Design review of the part built by this model. Coordinates are the model's own, in mm. A direction names the side the tool comes from. Give positions to 0.01 mm unless a question says otherwise; leave off trailing zeros. Order: outer loops, then holes, each group sorted by start corner. A loop starts at its lowest first (then second) coordinate and runs counter-clockwise, first axis right, second up. Notation, with made-up numbers: (61.5, 77.5) -> (119.5, 77.5) arc R13 cw to (119.5, 86.5) -> close; hole circle Ø11 at (31, 34.5). An arc over 180 degrees is marked (long way). Answer in a Markdown table with one row per item. Add a question column.
```python
from build123d import *

# Parameters (mm, degrees)
SKETCH1_W           = 110
SKETCH1_H           = 140
SKETCH1_R           = 2
SKETCH1_R_2         = 2.425
BOSS_EXTRUDE1_DEPTH = 10
FILLET1_R           = 10
SKETCH3_W           = 28.5
SKETCH3_H           = 55
CUT_EXTRUDE1_DEPTH  = 8
CHAMFER1_SIZE       = 8
SKETCH5_R           = 2
CUT_EXTRUDE3_DEPTH  = 8
CUT_EXTRUDE4_START  = -8
SKETCH6_R           = 2
CUT_EXTRUDE4_DEPTH  = 8
SKETCH7_W           = 110
SKETCH7_H           = 15
CUT_EXTRUDE7_DEPTH  = 2.5
CHAMFER3_SIZE       = 2.5
CHAMFER4_SIZE       = 1.5
CUT_EXTRUDE8_DEPTH  = 3
BOSS_EXTRUDE3_DEPTH = 10
SKETCH10_W          = 6.9
SKETCH10_H          = 6.9
CUT_EXTRUDE9_DEPTH  = 5
BOSS_EXTRUDE4_DEPTH = 10


with BuildPart() as part:
    # Sketch1 → Boss-Extrude1 (new body)
    with BuildSketch(Plane.XY):
        Rectangle(SKETCH1_W, SKETCH1_H)
        with Locations((-26.5, 50.75)):
            Circle(SKETCH1_R, mode=Mode.SUBTRACT)
        with Locations(Location((26.5, 50.75, 0), (0, 0, 180))):
            Circle(SKETCH1_R, mode=Mode.SUBTRACT)
        with Locations((26.5, -50.75)):
            Circle(SKETCH1_R, mode=Mode.SUBTRACT)
        with Locations(Location((-26.5, -50.75, 0), (0, 0, 180))):
            Circle(SKETCH1_R, mode=Mode.SUBTRACT)
        with Locations((-40, 55)):
            Circle(SKETCH1_R_2, mode=Mode.SUBTRACT)
        with Locations(Location((40, 55, 0), (0, 0, 180))):
            Circle(SKETCH1_R_2, mode=Mode.SUBTRACT)
        with Locations((40, -55)):
            Circle(SKETCH1_R_2, mode=Mode.SUBTRACT)
        with Locations(Location((-40, -55, 0), (0, 0, 180))):
            Circle(SKETCH1_R_2, mode=Mode.SUBTRACT)
        with Locations((-39.8, 49)):
            Circle(SKETCH1_R_2, mode=Mode.SUBTRACT)
        with Locations(Location((39.8, 49, 0), (0, 0, 180))):
            Circle(SKETCH1_R_2, mode=Mode.SUBTRACT)
        with Locations((39.8, -49)):
            Circle(SKETCH1_R_2, mode=Mode.SUBTRACT)
        with Locations(Location((-39.8, -49, 0), (0, 0, 180))):
            Circle(SKETCH1_R_2, mode=Mode.SUBTRACT)
        with Locations((-39.6, 43.00333426)):
            Circle(SKETCH1_R_2, mode=Mode.SUBTRACT)
        with Locations(Location((39.6, 43.00333426, 0), (0, 0, 180))):
            Circle(SKETCH1_R_2, mode=Mode.SUBTRACT)
        with Locations((39.6, -43.00333426)):
            Circle(SKETCH1_R_2, mode=Mode.SUBTRACT)
        with Locations(Location((-39.6, -43.00333426, 0), (0, 0, 180))):
            Circle(SKETCH1_R_2, mode=Mode.SUBTRACT)
        with BuildLine():
            Line((-7.75, 40), (-7.75, 5))
            ThreePointArc((-7.75, 5), (-9, 3.75), (-10.25, 5))
            Line((-10.25, 5), (-10.25, 40))
            ThreePointArc((-10.25, 40), (-9, 41.25), (-7.75, 40))
        make_face(mode=Mode.SUBTRACT)
        with BuildLine():
            Line((7.75, 40), (7.75, 5))
            ThreePointArc((7.75, 5), (9, 3.75), (10.25, 5))
            Line((10.25, 5), (10.25, 40))
            ThreePointArc((10.25, 40), (9, 41.25), (7.75, 40))
        make_face(mode=Mode.SUBTRACT)
    extrude(amount=BOSS_EXTRUDE1_DEPTH)

    # Fillet1
    fillet1_edges = [part.edges().sort_by_distance(p)[0] for p in [
        (55, -70, 5),
        (-55, -70, 5),
        (-55, 70, 5),
        (55, 70, 5),
    ]]
    fillet(fillet1_edges, radius=FILLET1_R)

    # Sketch3 → Cut-Extrude1 (cut)
    with BuildSketch(Plane.XY.offset(10)):
        with Locations((0, 22.5)):
            Rectangle(SKETCH3_W, SKETCH3_H)
    extrude(amount=-CUT_EXTRUDE1_DEPTH, mode=Mode.SUBTRACT)

    # Chamfer1
    chamfer1_edges = [part.edges().sort_by_distance(p)[0] for p in [
        (0, -5, 10),
        (14.25, 22.5, 10),
        (0, 50, 10),
        (-14.25, 22.5, 10),
    ]]
    chamfer(chamfer1_edges, length=CHAMFER1_SIZE - 0.0001)  # a hair under: the kernel refuses the full size

    # Sketch5 → Cut-Extrude3 (cut)
    with BuildSketch(Plane.ZY.offset(55)):
        with Locations(Location((5, 50, 0), (0, 0, 270))):
            Circle(SKETCH5_R)
        with Locations(Location((5, 40, 0), (0, 0, 270))):
            Circle(SKETCH5_R)
        with Locations(Location((5, 30, 0), (0, 0, 270))):
            Circle(SKETCH5_R)
        with Locations(Location((5, 20, 0), (0, 0, 270))):
            Circle(SKETCH5_R)
        with Locations(Location((5, 10, 0), (0, 0, 270))):
            Circle(SKETCH5_R)
        with Locations(Location((5, 0, 0), (0, 0, 270))):
            Circle(SKETCH5_R)
        with Locations(Location((5, -10, 0), (0, 0, 270))):
            Circle(SKETCH5_R)
        with Locations(Location((5, -20, 0), (0, 0, 270))):
            Circle(SKETCH5_R)
        with Locations(Location((5, -30, 0), (0, 0, 270))):
            Circle(SKETCH5_R)
        with Locations(Location((5, -40, 0), (0, 0, 270))):
            Circle(SKETCH5_R)
        with Locations(Location((5, -50, 0), (0, 0, 270))):
            Circle(SKETCH5_R)
    extrude(amount=-CUT_EXTRUDE3_DEPTH, mode=Mode.SUBTRACT)

    # Sketch6 → Cut-Extrude4 (cut)
    with BuildSketch(Plane(origin=(55, 0, 0), x_dir=(0, 0, -1), z_dir=(1, 0, 0)).offset(CUT_EXTRUDE4_START)):
        with Locations(Location((-5, 50, 0), (0, 0, 270))):
            Circle(SKETCH6_R)
        with Locations(Location((-5, 40, 0), (0, 0, 270))):
            Circle(SKETCH6_R)
        with Locations(Location((-5, 30, 0), (0, 0, 270))):
            Circle(SKETCH6_R)
        with Locations(Location((-5, 20, 0), (0, 0, 270))):
            Circle(SKETCH6_R)
        with Locations(Location((-5, 10, 0), (0, 0, 270))):
            Circle(SKETCH6_R)
        with Locations(Location((-5, 0, 0), (0, 0, 270))):
            Circle(SKETCH6_R)
        with Locations(Location((-5, -10, 0), (0, 0, 270))):
            Circle(SKETCH6_R)
        with Locations(Location((-5, -20, 0), (0, 0, 270))):
            Circle(SKETCH6_R)
        with Locations(Location((-5, -30, 0), (0, 0, 270))):
            Circle(SKETCH6_R)
        with Locations(Location((-5, -40, 0), (0, 0, 270))):
            Circle(SKETCH6_R)
        with Locations(Location((-5, -50, 0), (0, 0, 270))):
            Circle(SKETCH6_R)
    extrude(amount=CUT_EXTRUDE4_DEPTH, mode=Mode.SUBTRACT)

    # Sketch7 → Cut-Extrude7 (cut)
    with BuildSketch(Plane.XY.offset(10)):
        with Locations((0, -15.5)):
            Rectangle(SKETCH7_W, SKETCH7_H)
    extrude(amount=-CUT_EXTRUDE7_DEPTH, mode=Mode.SUBTRACT)

    # Chamfer3
    chamfer3_edges = [part.edges().sort_by_distance(p)[0] for p in [
        (0, -23, 7.5),
        (-37.37495, -8, 7.5),
        (37.37495, -8, 7.5),
    ]]
    chamfer(chamfer3_edges, length=CHAMFER3_SIZE - 0.0001)  # a hair under: the kernel refuses the full size

    # Chamfer4
    chamfer4_edges = [part.edges().sort_by_distance(p)[0] for p in [
        (0, -70, 0),
        (0, -70, 10),
        (55, 0, 0),
        (-55, 0, 0),
        (0, 70, 0),
        (52.071067812, 67.071067812, 0),
        (-52.071067812, 67.071067812, 0),
        (52.071067812, -67.071067812, 0),
        (-52.071067812, -67.071067812, 0),
        (-55, 26, 10),
        (55, -41.5, 10),
        (0, 70, 10),
        (52.071067812, 67.071067812, 10),
        (-52.071067812, 67.071067812, 10),
        (52.071067812, -67.071067812, 10),
        (-52.071067812, -67.071067812, 10),
        (-55, -41.5, 10),
        (55, 26, 10),
    ]]
    chamfer(chamfer4_edges, length=CHAMFER4_SIZE)

    # Sketch8 → Cut-Extrude8 (cut)
    with BuildSketch(Plane(origin=(0, 0, 10), x_dir=(-1, 0, 0), z_dir=(0, 0, -1))):
        with BuildLine():
            Line((-45.8, 43), (-45.8, 55))
            ThreePointArc((-45.8, 55), (-39.8, 61), (-33.8, 55))
            Line((-33.8, 55), (-33.8, 43))
            ThreePointArc((-33.8, 43), (-39.8, 37), (-45.8, 43))
        make_face()
        with BuildLine():
            Line((45.8, 43), (45.8, 55))
            ThreePointArc((45.8, 55), (39.8, 61), (33.8, 55))
            Line((33.8, 55), (33.8, 43))
            ThreePointArc((33.8, 43), (39.8, 37), (45.8, 43))
        make_face()
        with BuildLine():
            Line((45.8, -43), (45.8, -55))
            ThreePointArc((45.8, -55), (39.8, -61), (33.8, -55))
            Line((33.8, -55), (33.8, -43))
            ThreePointArc((33.8, -43), (39.8, -37), (45.8, -43))
        make_face()
        with BuildLine():
            Line((-45.8, -43), (-45.8, -55))
            ThreePointArc((-45.8, -55), (-39.8, -61), (-33.8, -55))
            Line((-33.8, -55), (-33.8, -43))
            ThreePointArc((-33.8, -43), (-39.8, -37), (-45.8, -43))
        make_face()
    extrude(amount=CUT_EXTRUDE8_DEPTH, mode=Mode.SUBTRACT)

    # Sketch9 → Boss-Extrude3 (add)
    with BuildSketch(Plane(origin=(55, 0, 0), x_dir=(0, 0, -1), z_dir=(1, 0, 0))):
        Polygon((-7.479483029, -9.130730638), (-5.687930895, -6.827306465), (-2.453830288, -7.571847612), (-2.453830288, -22.439403639), (-6.432472041, -22.439403639), (-7.150561873, -20.576942606), (-7.150561873, -10.503478378), align=None)
    extrude(amount=-BOSS_EXTRUDE3_DEPTH)

    # Sketch10 → Cut-Extrude9 (cut)
    with BuildSketch(Plane(origin=(0, 0, 0), x_dir=(-1, 0, 0), z_dir=(0, 0, -1))):
        with Locations((-26.5, 50.75)):
            Rectangle(SKETCH10_W, SKETCH10_H)
        with Locations((26.5, 50.75)):
            Rectangle(SKETCH10_W, SKETCH10_H)
        with Locations((26.5, -50.75)):
            Rectangle(SKETCH10_W, SKETCH10_H)
        with Locations((-26.5, -50.75)):
            Rectangle(SKETCH10_W, SKETCH10_H)
    extrude(amount=-CUT_EXTRUDE9_DEPTH, mode=Mode.SUBTRACT)

    # Sketch11 → Boss-Extrude4 (add)
    with BuildSketch(Plane.ZY.offset(55)):
        Polygon((2.460121708, -8.614116327), (4.352652236, -6.895389623), (7.133513419, -6.895389623), (7.925286395, -8.961723975), (7.133513419, -10.622516071), (7.133513419, -21.398353157), (5, -22.866029893), (2.711171676, -22.614979925), (2.267006348, -15.044857814), align=None)
    extrude(amount=-BOSS_EXTRUDE4_DEPTH)


solid = part.part
```
1) Add section A-A, the plane y = 10. Give the number of separate pieces and of enclosed holes in the cut face, and give its area (4 significant figures).
2) Add section C-C, the plane y = -30. Write out the cut boundary in (x, z), and give its area (3 significant figures).
3) Mouldability with a two-part tool opening along X and no side actions: class faces 5 (the face through (-39.9, 61, 8.5)), 6 (the face through (55, -1, 3)), 7 (the face through (-1, -70, 5)) as +X half, -X half, draft (parallel to the pull), parting line (faces both ways), or undercut.
4) For L1, parallel to X at y = -49, z = 3 (3 decimals); L2, parallel to Y at x = -8.5, z = 4.75; L3, parallel to Y at x = -26.5, z = 6.3, list the stretches that pass through material, from the lowest coordinate up.
5) Machinability: for faces 1 (the face through (39.7, -37, 8.5)), 2 (the face through (-28, 52.3, 5)), 3 (the face through (51, 52, 5)), 4 (the face through (-51, 12, 5)), which of the approach directions +Z, -Z, +X, -X, +Y, -Y give a long, thin tool a straight path to every point of the face, cutting with its end or side? Answer none if there is none.
6) Clearance check with flat-ended pins moving along their axes: P1, Ø2.5, axis at y = 10, z = 5, coming from the -X side; P2, Ø3, axis at x = 3.5, y = -16.5, coming from the +Z side; P3, Ø9.5, axis at x = 40, y = 46.5, coming from the +Z side. State where each tip first meets the part, or that it passes through.
Verdict:
| question | item | result |
|---|---|---|
| 1 | separate pieces | 3 |
| 1 | enclosed holes | 0 |
| 1 | area | 729.5 mm2 |
| 2 | outline | (-55, 1.5) -> (-53.5, 0) -> (53.5, 0) -> (55, 1.5) -> (55, 3) -> (47, 3) -> (47, 7) -> (55, 7) -> (55, 8.5) -> (53.5, 10) -> (-53.5, 10) -> (-55, 8.5) -> (-55, 7) -> (-47, 7) -> (-47, 3) -> (-55, 3) -> close |
| 2 | area | 1,030 mm2 |
| 3 | face 5 | undercut |
| 3 | face 6 | +X half |
| 3 | face 7 | draft |
| 4 | L1 | x = -55 to -42.225, -37.375 to -29.95, -23.05 to 23.05, 29.95 to 37.375, 42.225 to 55 |
| 4 | L2 | y = -70 to -7.75, 52.75 to 70 |
| 4 | L3 | y = -70 to -52.75, -48.75 to 48.75, 52.75 to 70 |
| 5 | face 1 | +Z |
| 5 | face 2 | -Z |
| 5 | face 3 | +X |
| 5 | face 4 | -X |
| 6 | P1 | stops at x = -47 |
| 6 | P2 | stops at z = 7.5 |
| 6 | P3 | stops at z = 7 |
